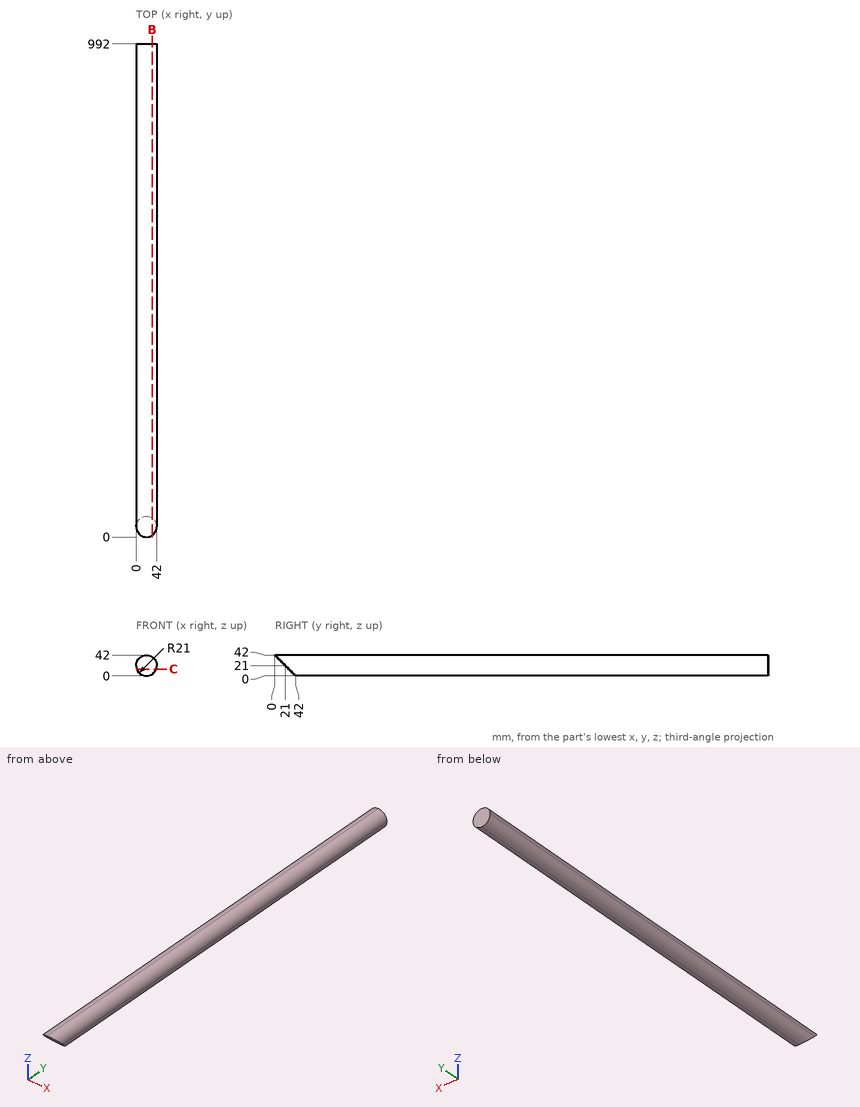
For this review, use the dimensioned drawing (mm, ordinates from the lowest corner) and the shaded views. Give positions to 0.01 mm unless a question says otherwise; leave off trailing zeros. Loops run counter-clockwise (first coordinate to the right, second up) from the corner with the lowest first, then second, coordinate; pieces in that order, holes last.
Item 1: For line 1 along X through (y, z) = (219.5, 18.5); line 2 along X through (y, z) = (429, 21.5); line 3 along Z through (x, y) = (38.5, 666.5), list the stretches that pass through material, from the lowest coordinate up.
Item 2: Take a section at C-C, the plane z = 14. State the section outline as (x, y) points, and give its area (3 significant figures).
Item 3: Take a section at B-B, the plane x = 32.5. State the section outline as (y, z) points.
Item 4: Insertion check: pin 1 (2 mm diameter, centred on x = 12.5, y = 347, fed in from +Z) (3 decimals); pin 2 (4 mm diameter, centred on x = 12, y = 883, fed in from +Z); pin 3 (2 mm diameter, centred on x = 14.5, y = 825.5, fed in from +Z). Each pin has a flat end and moves straight along its axis. Give the tip position at first contact, or say it passes through.
Calculated:
1. line 1: x = 0.15 to 41.85
1. line 2: x = 0.01 to 41.99
1. line 3: z = 9.39 to 32.61
2. outline: (1.2, 28) - (40.8, 28) - (40.8, 992) - (1.2, 992) - close
2. area: 38,200 mm2
3. outline: (3.43, 38.57) - (38.57, 3.43) - (992, 3.43) - (992, 38.57) - close
4. pin 1: stops at z = 40.615
4. pin 2: stops at z = 40.8
4. pin 3: stops at z = 41.27
